from build123d import *

# Parameters (mm, degrees)
EXTRUDE_1_DEPTH     = 12
SKETCH_2_R          = 1.75
CUT_EXTRUDE_1_DEPTH = 46.453272709
CUT_EXTRUDE_2_DEPTH = 2.5
FILLET_2_R          = 2
FILLET_3_R          = 1.5
FILLET_5_R          = 0.8
CHAMFER_2_SIZE      = 0.5


with BuildPart() as part:
    # 草图1 → 凸台-拉伸1 (new body)
    with BuildSketch(Plane.XY):
        with BuildLine():
            Line((4, 30.740852298), (-4, 30.740852298))
            ThreePointArc((-4, 30.740852298), (0, -31), (4, 30.740852298))
        make_face()
    extrude(amount=EXTRUDE_1_DEPTH)

    # 草图2 → 切除-拉伸1 (cut, through all)
    with BuildSketch(Plane.XY.offset(12)):
        with Locations((0, -12.5)):
            Circle(SKETCH_2_R)
    extrude(amount=-CUT_EXTRUDE_1_DEPTH, mode=Mode.SUBTRACT)

    # 草图4 → 切除-拉伸2 (cut)
    with BuildSketch(Plane.XY.offset(12)):
        with BuildLine():
            Line((14.60159577, -21.303320164), (6.823421177, -13.525145571))
            ThreePointArc((6.823421177, -13.525145571), (6.899952258, -12.525667942), (6.83085934, -11.525648589))
            Line((6.83085934, -11.525648589), (14.609033933, -3.747473996))
            ThreePointArc((14.609033933, -3.747473996), (14.67380701, 2.072232238), (8.853780377, 2.09382366))
            Line((8.853780377, 2.09382366), (1.075605784, -5.684350934))
            ThreePointArc((1.075605784, -5.684350934), (0.025527626, -5.600047222), (-1.025145571, -5.676578823))
            Line((-1.025145571, -5.676578823), (-8.803320164, 2.10159577))
            ThreePointArc((-8.803320164, 2.10159577), (-14.60159577, 2.10159577), (-14.60159577, -3.696679836))
            Line((-14.60159577, -3.696679836), (-6.823421177, -11.474854429))
            ThreePointArc((-6.823421177, -11.474854429), (-6.899952778, -12.525527626), (-6.815649066, -13.575605784))
            Line((-6.815649066, -13.575605784), (-14.59382366, -21.353780377))
            ThreePointArc((-14.59382366, -21.353780377), (-14.572232238, -27.17380701), (-8.752526004, -27.109033933))
            Line((-8.752526004, -27.109033933), (-0.974351411, -19.33085934))
            ThreePointArc((-0.974351411, -19.33085934), (0.025667942, -19.399952258), (1.025145571, -19.323421177))
            Line((1.025145571, -19.323421177), (8.803320164, -27.10159577))
            ThreePointArc((8.803320164, -27.10159577), (14.60159577, -27.10159577), (14.60159577, -21.303320164))
        make_face()
    extrude(amount=-CUT_EXTRUDE_2_DEPTH, mode=Mode.SUBTRACT)

    # 圆角2
    fillet_2_edges = [part.edges().sort_by_distance(p)[0] for p in [
        (-4, 30.740852298, 6),
        (4, 30.740852298, 6),
    ]]
    fillet(fillet_2_edges, radius=FILLET_2_R)

    # 圆角3
    # the kernel refuses this fillet: 1.5 mm, written as the material it takes off along each edge
    with BuildSketch(Plane(origin=(0, 0, 12), x_dir=(-0.5266668059049125, -0.8500718061187049, 0), z_dir=(-0.8500718061187049, 0.5266668059049125, 0))) as fillet_3_piece_1:
        with BuildLine():
            CenterArc((31 - FILLET_3_R, -FILLET_3_R), FILLET_3_R, 0, 90)
            Line((31, -FILLET_3_R), (31, 0))
            Line((31, 0), (31 - FILLET_3_R, 0))
        make_face()
    revolve(axis=Axis((0, 0, 12), (0, 0, 1)), revolution_arc=204.115094482, mode=Mode.SUBTRACT)
    with BuildSketch(Plane(origin=(3.868256609, 30.740852298, 0), x_dir=(0, 0, 1), z_dir=(-1, 0, 0))) as fillet_3_piece_2:
        with BuildLine():
            CenterArc((FILLET_3_R, -FILLET_3_R), FILLET_3_R, 90, 90)
            Line((0, -FILLET_3_R), (0, 0))
            Line((0, 0), (FILLET_3_R, 0))
        make_face()
    extrude(amount=7.736513218, mode=Mode.SUBTRACT)
    with BuildSketch(Plane(origin=(3.868256609, 30.740852298, 12), x_dir=(0, 0, -1), z_dir=(-1, 0, 0))) as fillet_3_piece_3:
        with BuildLine():
            CenterArc((FILLET_3_R, FILLET_3_R), FILLET_3_R, 180, 90)
            Line((0, FILLET_3_R), (0, 0))
            Line((0, 0), (FILLET_3_R, 0))
        make_face()
    extrude(amount=7.736513218, mode=Mode.SUBTRACT)
    with BuildSketch(Plane(origin=(0, 0, 0), x_dir=(-0.1333881589240954, 0.991063872340648, 0), z_dir=(0.991063872340648, 0.1333881589240954, 0))) as fillet_3_piece_4:
        with BuildLine():
            CenterArc((31 - FILLET_3_R, FILLET_3_R), FILLET_3_R, 270, 90)
            Line((31, FILLET_3_R), (31, 0))
            Line((31, 0), (31 - FILLET_3_R, 0))
        make_face()
    revolve(axis=Axis((0, 0, 0), (0, 0, 1)), revolution_arc=344.669149504, mode=Mode.SUBTRACT)
    with BuildSketch(Plane(origin=(-3.868256609, 28.740852298, 0), x_dir=(0, 1, 0), z_dir=(1, 0, 0))) as fillet_3_piece_5:
        with BuildLine():
            CenterArc((2 - FILLET_3_R, FILLET_3_R), FILLET_3_R, 270, 90)
            Line((2, FILLET_3_R), (2, 0))
            Line((2, 0), (2 - FILLET_3_R, 0))
        make_face()
    revolve(axis=Axis((-3.868256609, 28.740852298, 0), (0, 0, 1)), revolution_arc=7.665425248, mode=Mode.SUBTRACT)
    with BuildSketch(Plane(origin=(3.868256609, 28.740852298, 0), x_dir=(0, 1, 0), z_dir=(-1, 0, 0))) as fillet_3_piece_6:
        with BuildLine():
            CenterArc((2 - FILLET_3_R, -FILLET_3_R), FILLET_3_R, 0, 90)
            Line((2, -FILLET_3_R), (2, 0))
            Line((2, 0), (2 - FILLET_3_R, 0))
        make_face()
    revolve(axis=Axis((3.868256609, 28.740852298, 0), (0, 0, -1)), revolution_arc=7.665425248, mode=Mode.SUBTRACT)
    with BuildSketch(Plane(origin=(0, 0, 12), x_dir=(-0.1333881589240954, 0.991063872340648, 0), z_dir=(0.991063872340648, 0.1333881589240954, 0))) as fillet_3_piece_7:
        with BuildLine():
            CenterArc((31 - FILLET_3_R, -FILLET_3_R), FILLET_3_R, 0, 90)
            Line((31, -FILLET_3_R), (31, 0))
            Line((31, 0), (31 - FILLET_3_R, 0))
        make_face()
    revolve(axis=Axis((0, 0, 12), (0, 0, 1)), revolution_arc=152.623466515, mode=Mode.SUBTRACT)
    with BuildSketch(Plane(origin=(-3.868256609, 28.740852298, 12), x_dir=(0, 1, 0), z_dir=(1, 0, 0))) as fillet_3_piece_8:
        with BuildLine():
            CenterArc((2 - FILLET_3_R, -FILLET_3_R), FILLET_3_R, 0, 90)
            Line((2 - FILLET_3_R, 0), (2, 0))
            Line((2, 0), (2, -FILLET_3_R))
        make_face()
    revolve(axis=Axis((-3.868256609, 28.740852298, 12), (0, 0, 1)), revolution_arc=7.665425248, mode=Mode.SUBTRACT)
    with BuildSketch(Plane(origin=(3.868256609, 28.740852298, 12), x_dir=(0, 1, 0), z_dir=(-1, 0, 0))) as fillet_3_piece_9:
        with BuildLine():
            CenterArc((2 - FILLET_3_R, FILLET_3_R), FILLET_3_R, 270, 90)
            Line((2 - FILLET_3_R, 0), (2, 0))
            Line((2, 0), (2, FILLET_3_R))
        make_face()
    revolve(axis=Axis((3.868256609, 28.740852298, 12), (0, 0, -1)), revolution_arc=7.665425248, mode=Mode.SUBTRACT)

    # 圆角5
    fillet_5_edges = [part.edges().sort_by_distance(p)[0] for p in [
        (6.83085934, -11.525648589, 10.75),
        (6.823421177, -13.525145571, 10.75),
        (1.025145571, -19.323421177, 10.75),
        (-0.974351411, -19.33085934, 10.75),
        (-6.815649066, -13.575605784, 10.75),
        (-6.823421177, -11.474854429, 10.75),
        (-1.025145571, -5.676578823, 10.75),
        (1.075605784, -5.684350934, 10.75),
    ]]
    fillet(fillet_5_edges, radius=FILLET_5_R)

    # 倒角2
    chamfer_2_edges = [part.edges().sort_by_distance(p)[0] for p in [
        (-1.75, -12.5, 0),
        (-1.75, -12.5, 9.5),
    ]]
    chamfer(chamfer_2_edges, length=CHAMFER_2_SIZE)


solid = part.part
Model file for the job. Use its own axes, mm. A direction names the side the tool comes from. Give positions to 0.01 mm unless a question says otherwise; leave off trailing zeros. Write each loop counter-clockwise with the first axis right and the second up, starting at its lowest first coordinate (ties: lowest second). Pieces come first, ordered by that corner, then holes. Notation, with made-up numbers: (9.5, -7.5) - (39.5, -7.5) arc R18 cw to (39.5, 12.5) - close; hole circle Ø3 at (-23.5, 36). An arc over 180 degrees is marked (long way). Answer as CSV lines item,"result".
1. Two-plate mould, pull along X, no slides. Class faces 3 (the face through (0, -25, 12)), 4 (the face through (-1.305, -30.973, 5.937)), 5 (the face through (0, -5.6, 10.8)): +X half, -X half, draft (parallel to the pull), parting line (faces both ways), or undercut.
Responses:
face 3,"draft"
face 4,"parting line"
face 5,"undercut"
2. Band-saw the part on A-A (y = 0). Write the cut outline in (x, z), and give its area (3 significant figures).
Responses:
outline,"(-31, 1.5) arc R1.5 ccw to (-29.5, 0) - (29.5, 0) arc R1.5 ccw to (31, 1.5) - (31, 10.5) arc R1.5 ccw to (29.5, 12) - (15.77, 12) - (15.77, 9.5) - (6.76, 9.5) - (6.76, 12) - (-6.7, 12) - (-6.7, 9.5) - (-15.72, 9.5) - (-15.72, 12) - (-29.5, 12) arc R1.5 ccw to (-31, 10.5) - close"
area,"697 mm2"
3. Pin check, flat tips, straight feed: pin 1 (6 mm diameter, centred on y = -10, z = 3, fed in from +X); pin 2 (1.5 mm diameter, centred on x = 20, z = 6, fed in from -Y); pin 3 (1 mm diameter, centred on y = -19.5, z = 7.5, fed in from -X). Stop position of each tip, or through.
Responses:
pin 1,"stops at x = 30.2"
pin 2,"stops at y = -24.3"
pin 3,"stops at x = -24.49"
4. 3-axis set-ups, long thin cutter, end or side, ignore diameter. For faces 1 (the face through (14.737, 2.007, 10.768)), 2 (the face through (0.05, 30.31, 0.45)): which of +Z, -Z, +X, -X, +Y, -Y reach the whole face in a straight line?
Responses:
face 1,"+Z"
face 2,"-Z, +X, -X, +Y"
5. Drill centre lines: L1, parallel to Y at x = 0, z = 3; L2, parallel to Y at x = -23, z = 2.5; L3, parallel to Y at x = -12, z = 9. Where is each one in solid material? Low to high. Write a range as [from, to].
Responses:
L1,"y = [-31, -14.25], [-10.75, 30.74]"
L2,"y = [-20.78, 20.78]"
L3,"y = [-28.58, 28.58]"
